Part model, mm, in its own coordinate system. A direction names the side the tool comes from. Give positions to 0.01 mm unless a question says otherwise; leave off trailing zeros. Order: outer loops, then holes, each group sorted by start corner. A loop starts at its lowest first (then second) coordinate and runs counter-clockwise, first axis right, second up.
1. Slice it at D-D on z = -16.5. List the corners of the cut face in (x, y).
2. Drop flat-ended pins along their axis: pin 1 Ø6 at (x, y) = (22, 0) entering from -Z; pin 2 Ø2.5 at (x, y) = (37, -0.5) entering from -Z; pin 3 Ø1 at (x, y) = (-16.5, -1.5) entering from +Z; pin 4 Ø3 at (x, y) = (-12.5, -7) entering from +Z. Give the stop position or say it passes through.
3. Which spindle directions (+Z, -Z, +X, -X, +Y, -Y) get a long thin tool onto all of the face, cutting with end or side? Do faces 1 (the flat face through (-2, 1.5, -27)), 2 (the cylindrical face through (-25.27, 0.76, 16.17)), 3 (the flat face through (32.9, -2.5, 10.4)). Say none if no direction does.
4. Slice it at A-A on y = -13. List the corners of the cut face in (x, z).
5. Probe line 1 (Y direction, x = 37, z = 0); line 2 (Z direction, x = -36.6, y = -10); line 3 (X direction, y = 0.25, z = 26.5). List the from-to ranges inside material, lowest first.
6. Slice it at C-C on x = -24.5. List the corners of the cut face in (y, z), and give its area (3 significant figures).
7. Mould opens along X. For faces 4 (the flat face through (-37, -15, 0)), 5 (the cylindrical face through (15.734, -0.986, 16.084)), 6 (the flat face through (10.4, -2.5, 32.9)), 7 (the cylindrical face through (-15.377, -2.986, -16.426)) say: +X half, -X half, draft (parallel to the pull), parting line (faces both ways), or undercut.
8. Slice it at B-B on y = 4.75. List the corners of the cut face in (x, z), and give its area (3 significant figures).
Autodesk Inventor part; units mm, degrees
ref_plane "YZ Plane" through (0, 0, 0) normal (1, 0, 0) x (0, 1, 0)
ref_plane "XZ Plane" through (0, 0, 0) normal (0, 1, 0) x (-1, 0, 0)
ref_plane "XY Plane" through (0, 0, 0) normal (0, 0, 1) x (1, 0, 0)
sketch "Sketch1" plane through (0, 0, 0) normal (0, 1, 0) x (-1, 0, 0)
  circle A0 centre (0, 0) radius 26.25
  circle A1 centre (0, 0) radius 33
  dimension "d0" = 52.5
  dimension "d1" = 66
extrude "Extrusion1" add sketch "Sketch1" along normal blind 1.5
sketch "Sketch2" plane through (0, 1.5, 0) normal (0, 1, 0) x (1, 0, 0)
  circle A0 centre (0, 0) radius 25
  circle A1 centre (0, 0) radius 33
  line L0 (-7.5, -23.8485) -> (-13.6817, -30.0302)
  circle A2 centre (0, 0) radius 33
  line L1 (-7.5, -23.8485) -> (1.2422, -23.8485) construction
  line L2 (7.5, -23.8485) -> (13.6817, -30.0302)
  line L3 (7.5, -23.8485) -> (16.2422, -23.8485) construction
  point P0 (0, -25)
  dimension "d4" = 50
  dimension "d5" = 135
  dimension "d6" = 45
  dimension "d7" = 15
  dimension "d9" = 7.5
  dimension "d10" = 0
  dimension "d66" = 8
extrude "Extrusion2" cut sketch "Sketch2" against normal blind 1.5 contours A0 L2 A1 L0 picked at (9.3939, -28.7092)
sketch "Sketch3" plane through (0, 1.5, 0) normal (0, 1, 0) x (1, 0, 0)
  circle A0 centre (0, 0) radius 30
  arc A1 (13.6817, -30.0302) -> (-13.6817, -30.0302) centre (0, 0) ccw
  line L0 (8.4905, -24.839) -> (13.6817, -30.0302)
  line L1 (-30, -0.0025) -> (-33, -0.0025)
  arc A2 (13.6817, -30.0302) -> (-13.6817, -30.0302) centre (0, 0) ccw
  line L2 (-30, -0.0025) -> (-27, -0.0025) construction
  line L3 (-10.6624, -27.0109) -> (-13.6817, -30.0302)
  line L4 (13.6817, -30.0302) -> (8.4905, -24.839)
  line L5 (11.4008, -27.7493) -> (13.6817, -30.0302)
  line L6 (-8.4905, -24.839) -> (-13.6817, -30.0302)
  line L7 (-11.4008, -27.7493) -> (-13.6817, -30.0302)
  line L8 (30, -0.0025) -> (33, 0.0056)
  point P0 (7.5, -26.4575)
  point P1 (-7.5, -26.4575)
  dimension "d13" = 60
  dimension "d14" = 180
extrude "Extrusion3" cut sketch "Sketch3" against normal blind 10 contours A0 L3 A1 L1 | L8 A1 L0 A0
sketch "Sketch8" plane through (0, 0, 0) normal (0, -1, 0) x (1, 0, 0)
  circle A0 centre (0, 0) radius 33
  circle A1 centre (0, 0) radius 36
  dimension "d29" = 66
  dimension "d30" = 3
  dimension "d91" = 72
extrude "Extrusion8" add sketch "Sketch8" against normal blind 6.5
sketch "Sketch16" plane through (0, 0, 0) normal (0, -1, 0) x (1, 0, 0)
  circle A0 centre (0, 0) radius 26.25
  dimension "d67" = 52.5
extrude "Extrusion13" add sketch "Sketch16" against normal blind 6.5
sketch "Sketch19" plane through (0, 6.5, 0) normal (0, 1, 0) x (1, 0, 0)
  circle A0 centre (0, 0) radius 24
  circle A1 centre (0, 0) radius 33
  line L0 (-7.5, -22.798) -> (-14.3681, -29.6661)
  circle A2 centre (0, 0) radius 32.9624
  line L1 (-7.5, -22.798) -> (2.213, -22.798) construction
  line L2 (7.5, -22.798) -> (14.3681, -29.6661)
  line L3 (7.5, -22.798) -> (17.213, -22.798) construction
  point P0 (0, -24)
  dimension "d70" = 48
  dimension "d71" = 135
  dimension "d72" = 45
  dimension "d73" = 15
  dimension "d74" = 7.5
  dimension "d75" = 0
  dimension "d76" = 9
  dimension "d138" = 66
extrude "Extrusion14" cut sketch "Sketch19" against normal blind 6.5 contours A0 L2 A2 L0 picked at (9.7463, -28.1973)
sketch "Sketch20" plane through (0, 0, 0) normal (0, -1, 0) x (1, 0, 0)
  circle A0 centre (0, 0) radius 36
  circle A1 centre (0, 0) radius 33
  dimension "d81" = 72
  dimension "d82" = 3
  dimension "d134" = 66
extrude "Extrusion15" add sketch "Sketch20" along normal blind 5
thread "Thread1"
sketch "Sketch21" plane through (0, 0, 0) normal (0, -1, 0) x (1, 0, 0)
  circle A0 centre (0, 0) radius 22.5
  circle A1 centre (0, 0) radius 23.5
  dimension "d87" = 45
  dimension "d88" = 1
extrude "Extrusion16" add sketch "Sketch21" along normal blind 4
sketch "Sketch23" plane through (0, 0, 0) normal (0, -1, 0) x (1, 0, 0)
  circle A0 centre (0, 0) radius 22.5
  line L0 (22.5, 0) -> (0, 22.5)
  line L1 (0, 22.5) -> (20.147, 42.647)
  line L2 (22.5, 0) -> (42.647, 20.147)
  line L3 (42.647, 20.147) -> (20.147, 42.647)
extrude "Extrusion17" cut sketch "Sketch23" along normal blind 5 contours A0 L1 L3 L2
sketch "Sketch24" plane through (0, 0, 0) normal (0, -1, 0) x (1, 0, 0)
  circle A0 centre (0, 0) radius 22.5
  dimension "d96" = 45
extrude "Extrusion18" add sketch "Sketch24" along normal blind 2
sketch "Sketch25" plane through (0, -5, 0) normal (0, -1, 0) x (1, 0, 0)
  line L0 (0, -5) -> (0, 5)
  line L1 (0, -5) -> (38, -5)
  line L2 (0, 5) -> (38, 5)
  line L3 (38, -5) -> (38, 5)
  circle A0 centre (0, 0) radius 36
  line L4 (0, -5) -> (-38, -5)
  line L5 (0, 5) -> (-38, 5)
  line L6 (-38, 5) -> (-38, -5)
  point P0 (35.6511, -5)
  point P1 (35.6511, 5)
  point P2 (-35.6511, -5)
  point P3 (-35.6511, 5)
  dimension "d99" = 10
  dimension "d100" = 5
  dimension "d101" = 38
  dimension "d102" = 38
  dimension "d107" = 38
  dimension "d133" = 72
extrude "Extrusion19" add sketch "Sketch25" along normal blind 10 and the other way blind 11.5 contours A0 L2 L3 L1 | L4 L6 L5 A0
sketch "Sketch26" plane through (38, -15, 5) normal (1, 0, 0) x (0, 0, -1)
  circle A0 centre (5, 5) radius 1.5
  line L0 (10, 0) -> (0, 0)
  line L1 (0, 10) -> (10, 10)
  line L2 (0, 10) -> (0, 0)
  line L3 (0, 21.5) -> (10, 21.5)
  point P0 (5, 15)
  dimension "d108" = 3
  dimension "d110" = 10
  dimension "d112" = 5
  dimension "d132" = 5
  dimension "d135" = 16.5
  dimension "d136" = 21.5
  dimension "d137" = 5
hole "Hole3" at (38, -10, 0) direction (-1, 0, 0) diameter 3 depth 8 tip angle 118
sketch "Sketch27" plane through (-38, -15, -5) normal (-1, 0, 0) x (0, 0, 1)
  line L0 (10, 0) -> (0, 0)
  line L1 (0, 10) -> (10, 10)
  circle A0 centre (5, 5) radius 1.5
  line L2 (10, 21.5) -> (10, 0)
  line L3 (0, 0) -> (0, 21.5)
  point P0 (5, 15)
  dimension "d120" = 10
  dimension "d121" = 3
  dimension "d122" = 5
  dimension "d123" = 10
  dimension "d124" = 5
hole "Hole4" at (-38, -10, 0) direction (1, 0, 0) diameter 3 depth 8 tip angle 118
equation "\"d102\" = d101"
equation "\"d107\" = d101"
properties part number "clock_case2"
Data:
1. outline: (-32, -5) - (-28.58, -5) - (-28.58, 0) - (-16.73, 0) - (-16.73, -4) - (-15.3, -4) - (-15.3, -2) - (15.3, -2) - (15.3, -4) - (16.73, -4) - (16.73, 0) - (28.58, 0) - (28.58, -5) - (32, -5) - (32, 6.5) - (28.58, 6.5) - (28.58, 1.5) - (20.42, 1.5) - (20.42, 6.5) - (-20.42, 6.5) - (-20.42, 1.5) - (-28.58, 1.5) - (-28.58, 6.5) - (-32, 6.5) - close
2. pin 1: stops at z = -30.58
2. pin 2: stops at z = -5
2. pin 3: stops at z = 32.25
2. pin 4: passes through
3. face 1: +Y
3. face 2: +Y, -Y
3. face 3: +Z, -Y
4. outline: (-38, -5) - (-35.65, -5) arc R36 cw to (-35.65, 5) - (-38, 5) - close; (35.65, -5) - (38, -5) - (38, 5) - (35.65, 5) arc R36 cw to start
5. line 1: y = -15 to -11.5, -8.5 to 6.5
5. line 2: z = -5 to -1.5, 1.5 to 5
5. line 3: x = -24.37 to -19.67, -14.06 to -11.2, 11.2 to 14.06, 19.67 to 24.37
6. outline: (-5, -26.38) - (6.5, -26.38) - (6.5, -22.11) - (1.5, -22.11) - (1.5, -9.42) - (6.5, -9.42) - (6.5, 9.42) - (1.5, 9.42) - (1.5, 17.31) - (0, 17.31) - (0, -22.11) - (-5, -22.11) - close; (-5, 22.11) - (6.5, 22.11) - (6.5, 26.38) - (-5, 26.38) - close
6. area: 252 mm2
7. face 4: draft
7. face 5: undercut
7. face 6: +X half
7. face 7: undercut
8. outline: (-38, -5) - (-35.65, -5) arc R36 ccw to (35.65, -5) - (38, -5) - (38, 5) - (35.65, 5) arc R36 ccw to (-35.65, 5) - (-38, 5) - close; (-9.26, 24.56) arc R26.25 ccw (long way) to (9.26, 24.56) - (7.5, 22.8) arc R24 ccw to (-7.5, 22.8) - close; hole circle Ø66 at (0, 0)
8. area: 2,820 mm2
